Here's how the part is built. I have some questions about the finished solid (model axes, mm). Face numbers are marked on the shaded views. A direction names the side the tool comes from. Round coordinates to 2 decimals unless told otherwise and drop trailing zeros. Write each loop counter-clockwise with the first axis right and the second up, starting at its lowest first coordinate (ties: lowest second). Pieces come first, ordered by that corner, then holes. Notation, with made-up numbers: (66.5, 85) -> (113.5, 85) arc R27 ccw to (113.5, 105) -> close; hole circle Ø5 at (4, 42). An arc over 180 degrees is marked (long way). Answer in a Markdown table with one row per item. Add a question column.
from build123d import *

# Parameters (mm, degrees)
F1_DEPTH = 2.54
F0_R     = 2.2225
F2_DEPTH = 19.05
F0_W     = 25.4
F0_H     = 25.4
F0_W_2   = 6.8400954445
F0_H_2   = 6.9419826217
F3_DEPTH = 25.4


with BuildPart() as f1:
    # F0 (on Top) → F1 (new body)
    with BuildSketch(Plane.XY):
        Polygon((16.1757896501, -1.1124916385), (16.1757896501, 7.8635431181), (9.3356942055, 7.8635431181), (9.3356942055, 14.8055257398), (0.1558850946, 14.8055257398), (0.1558850946, 7.8635431181), (-6.6842103499, 7.8635431181), (-6.6842103499, -1.1124916385), (0.1558850946, -1.1124916385), (0.1558850946, -8.0544742602), (9.3356942055, -8.0544742602), (9.3356942055, -1.1124916385), align=None)
    extrude(amount=F1_DEPTH)



with BuildPart() as f2:
    # F0 (on Top) → F2 (new body)
    with BuildSketch(Plane.XY):
        with Locations((-3.5092103499, 11.6305257398)):
            Circle(F0_R)
    extrude(amount=F2_DEPTH)


with BuildPart() as f2b:
    # F0 (on Top) → F2, piece 2 (new body)
    with BuildSketch(Plane.XY):
        with Locations((13.0007896501, 11.6305257398)):
            Circle(F0_R)
    extrude(amount=F2_DEPTH)


with BuildPart() as f2c:
    # F0 (on Top) → F2, piece 3 (new body)
    with BuildSketch(Plane.XY):
        with Locations((13.0007896501, -4.8794742602)):
            Circle(F0_R)
    extrude(amount=F2_DEPTH)


with BuildPart() as f2d:
    # F0 (on Top) → F2, piece 4 (new body)
    with BuildSketch(Plane.XY):
        with Locations((-3.5092103499, -4.8794742602)):
            Circle(F0_R)
    extrude(amount=F2_DEPTH)


with BuildPart() as f1_1:
    add(f1.part)

    add(f2.part)  # F3 merges F2

    add(f2b.part)  # F3 merges F2b

    add(f2c.part)  # F3 merges F2c

    add(f2d.part)  # F3 merges F2d
    # F0 (on Top) → F3 (join)
    with BuildSketch(Plane.XY):
        with Locations((4.7457896501, 3.3755257398)):
            Rectangle(F0_W, F0_H)
        Polygon((13.6357896501, 14.8055257398), (16.1757896501, 14.8055257398), (16.1757896501, 7.8635431181), (16.1757896501, -1.1124916385), (16.1757896501, -8.0544742602), (9.3356942055, -8.0544742602), (0.1558850946, -8.0544742602), (-4.1442103499, -8.0544742602), (-6.6842103499, -8.0544742602), (-6.6842103499, -1.1124916385), (-6.6842103499, 7.8635431181), (-6.6842103499, 14.8055257398), (-4.1442103499, 14.8055257398), (0.1558850946, 14.8055257398), (9.3356942055, 14.8055257398), align=None, mode=Mode.SUBTRACT)
        Polygon((0.1558850946, 7.8635431181), (0.1558850946, 14.8055257398), (-4.1442103499, 14.8055257398), (-6.6842103499, 14.8055257398), (-6.6842103499, 7.8635431181), align=None)
        with Locations((-3.5092103499, 11.6305257398)):
            Circle(F0_R, mode=Mode.SUBTRACT)
        Polygon((-4.1442103499, -8.0544742602), (0.1558850946, -8.0544742602), (0.1558850946, -1.1124916385), (-6.6842103499, -1.1124916385), (-6.6842103499, -8.0544742602), align=None)
        with Locations((-3.5092103499, -4.8794742602)):
            Circle(F0_R, mode=Mode.SUBTRACT)
        with Locations((12.7557419278, -4.5834829494)):
            Rectangle(F0_W_2, F0_H_2)
        with Locations((13.0007896501, -4.8794742602)):
            Circle(F0_R, mode=Mode.SUBTRACT)
        Polygon((16.1757896501, 7.8635431181), (16.1757896501, 14.8055257398), (13.6357896501, 14.8055257398), (9.3356942055, 14.8055257398), (9.3356942055, 7.8635431181), align=None)
        with Locations((13.0007896501, 11.6305257398)):
            Circle(F0_R, mode=Mode.SUBTRACT)
    extrude(amount=F3_DEPTH)


solid = f1_1.part
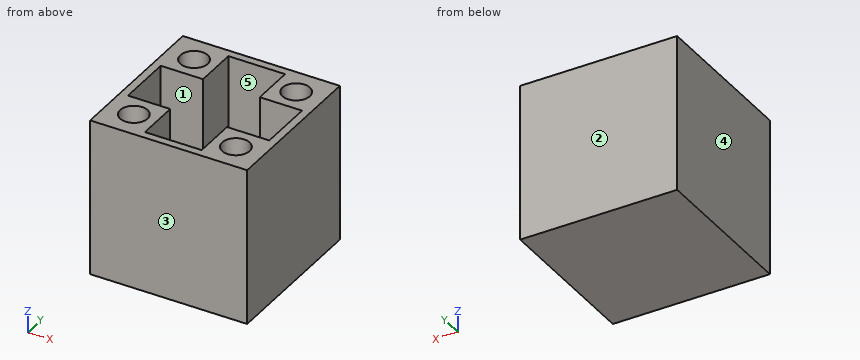
Item 1: I need wall thicknesses on line 1 along X through (y, z) = (13, 8.5); line 2 along X through (y, z) = (-0.25, 15.75); line 3 along Y through (x, z) = (9.75, 13.75). Which ranges of each line are inside material? Lowest first, please. Write a range as from..to.
Item 2: If we section it at B-B on x = 2.25: Please give me the cut outline in (y, z).
Item 3: If we mould it in two halves opening along X, with no side actions, what happens to the marked faces 3, 4 and 5? For each: pulls with the +X half, pulls with the -X half, needs draft (parallel to the pull), parting line crosses it, or undercut.
Item 4: If we section it at C-C on y = -0.5: Please give me the cut outline in (x, z).
Item 5: On a 3-axis mill with a long thin cutter (end or side, diameter ignored), from which of +Z, -Z, +X, -X, +Y, -Y can I reach the whole of each face in a straight line? I mean the marked faces 1 and 2. Say none if no direction works.
Item 6: If we section it at A-A on z = 8.5: Please give me the cut outline in (x, y).
Item 7: For P1, Ø1.3, axis at x = -4.5, y = -5, coming from the +Z side; P2, Ø6, axis at x = 13, y = 11.63, coming from the +Z side; P3, Ø11.5, axis at x = 4.5, y = 3, coming from the +Z side, each with a flat end and sliding along its axis, tell me the tip position at first contact or that it passes through.
Item 8: If we section it at D-D on z = 21.75: Please give me the cut outline in (x, y) (1 decimal).
Results list:
| question | item | result |
|---|---|---|
| 1 | line 1 | -7.95..0.16, 9.34..17.45 |
| 1 | line 2 | -7.95..-6.68, 16.18..17.45 |
| 1 | line 3 | -9.32..-1.11, 7.86..16.08 |
| 2 | outline | (-9.32, 0) -> (16.08, 0) -> (16.08, 25.4) -> (14.81, 25.4) -> (14.81, 2.54) -> (-8.05, 2.54) -> (-8.05, 25.4) -> (-9.32, 25.4) -> close |
| 3 | face 3 | needs draft |
| 3 | face 4 | pulls with the -X half |
| 3 | face 5 | undercut |
| 4 | outline | (-7.95, 0) -> (17.45, 0) -> (17.45, 25.4) -> (16.18, 25.4) -> (16.18, 2.54) -> (-6.68, 2.54) -> (-6.68, 25.4) -> (-7.95, 25.4) -> close |
| 5 | face 1 | +Z |
| 5 | face 2 | +Z, -Z, +X, -X, +Y |
| 6 | outline | (-7.95, -9.32) -> (17.45, -9.32) -> (17.45, 16.08) -> (-7.95, 16.08) -> close; hole (-6.68, -1.11) -> (0.16, -1.11) -> (0.16, -8.05) -> (9.34, -8.05) -> (9.34, -1.11) -> (16.18, -1.11) -> (16.18, 7.86) -> (9.34, 7.86) -> (9.34, 14.81) -> (0.16, 14.81) -> (0.16, 7.86) -> (-6.68, 7.86) -> close |
| 7 | P1 | z = 19.05 |
| 7 | P2 | z = 25.4 |
| 7 | P3 | z = 2.54 |
| 8 | outline | (-8, -9.3) -> (17.4, -9.3) -> (17.4, 16.1) -> (-8, 16.1) -> close; hole (-6.7, -1.1) -> (0.2, -1.1) -> (0.2, -8.1) -> (9.3, -8.1) -> (9.3, -1.1) -> (16.2, -1.1) -> (16.2, 7.9) -> (9.3, 7.9) -> (9.3, 14.8) -> (0.2, 14.8) -> (0.2, 7.9) -> (-6.7, 7.9) -> close; hole circle Ø4.4 at (-3.5, -4.9); hole circle Ø4.4 at (-3.5, 11.6); hole circle Ø4.4 at (13, -4.9); hole circle Ø4.4 at (13, 11.6) |
